Part model, mm, in its own coordinate system. A direction names the side the tool comes from. Round coordinates to 2 decimals unless told otherwise and drop trailing zeros. Loops run counter-clockwise (first coordinate to the right, second up) from the corner with the lowest first, then second, coordinate; pieces in that order, holes last.
(1) Cut at A-A on x = 0. List the corners of the cut face in (y, z), then the cut area to 3 significant figures.
(2) Probe probe 1 along X at (y, z) = (0, -12.5); probe 2 along Z at (x, y) = (7.6, 0). List the from-to ranges inside material, lowest first.
(3) Cut at B-B on z = -7. List the corners of the cut face in (x, y), then the cut area to 3 significant figures.
(4) Mould opens along Y. For faces 1 (the face through (7.829, 0.222, -2.875)), 2 (the face through (-1.9, 6.3, -15)), 3 (the face through (-8.82, 2.78, -7.9)) say: +Y half, -Y half, draft (parallel to the pull), parting line (faces both ways), or undercut.
(5) Tool access for faces 4 (the face through (-11.9, 3.7, 2.5)), 5 (the face through (9, -6, 0)): list every direction of +Z, -Z, +X, -X, +Y, -Y with a clear straight run to the whole face (end or side of a thin tool).
(6) Flat gauge pins, fed straight in: pin 1 (1.5 mm diameter, centred on x = 6.5, z = -6.5, fed in from +Y); pin 2 (8 mm diameter, centred on x = 7.5, z = -11, fed in from +Y); pin 3 (7 mm diameter, centred on x = 1, y = 4.5, fed in from -Z); pin 4 (0.9 mm diameter, centred on y = 0, z = -2.17, fed in from +X). Where does each tip first touch, or does it go through?
from build123d import *

# Parameters (mm, degrees)
SKETCH1_R           = 12.461427854
BASE_EXTRUDE_DEPTH  = 5
SKETCH2_R           = 9.246210184
BOSS_EXTRUDE1_DEPTH = 15
SKETCH3_W           = 6.4135
SKETCH3_H           = 13.726679844
SKETCH4_W           = 2.875338505
SKETCH4_H           = 0.738225097
SKETCH5_W           = 2.875338506
SKETCH5_H           = 0.738225097
FILLET1_R           = 1


with BuildPart() as part:
    # Sketch1 → Base-Extrude (new body)
    with BuildSketch(Plane(origin=(0, 0, 0), x_dir=(-1, 0, 0), z_dir=(0, 0, -1))):
        Circle(SKETCH1_R)
    extrude(amount=-BASE_EXTRUDE_DEPTH)

    # Sketch2 → Boss-Extrude1 (add)
    with BuildSketch(Plane(origin=(0, 0, 0), x_dir=(-1, 0, 0), z_dir=(0, 0, -1))):
        Circle(SKETCH2_R)
    extrude(amount=BOSS_EXTRUDE1_DEPTH)

    # Sketch3 → Cut-Revolve1 (revolve, cut)
    with BuildSketch(Plane.XZ):
        with Locations((3.20675, -8.136660078)):
            Rectangle(SKETCH3_W, SKETCH3_H)
    revolve(axis=Axis((0, 0, -1.273320156), (0, 0, -1)), mode=Mode.SUBTRACT)

    # Sketch4 → Cut-Revolve2 (revolve, cut)
    with BuildSketch(Plane(origin=(0, 0, 0), x_dir=(1, 0, 0), z_dir=(0, 1, 0))):
        with Locations((-7.808540932, 2.539892603)):
            Rectangle(SKETCH4_W, SKETCH4_H)
    revolve(axis=Axis((-9.246210184, 0, -2.170780054), (1, 0, 0)), mode=Mode.SUBTRACT)

    # Sketch5 → Cut-Revolve3 (revolve, cut)
    with BuildSketch(Plane(origin=(0, 0, 0), x_dir=(1, 0, 0), z_dir=(0, 1, 0))):
        with Locations((7.808540932, 2.539892603)):
            Rectangle(SKETCH5_W, SKETCH5_H)
    revolve(axis=Axis((6.370871679, 0, -2.170780054), (1, 0, 0)), mode=Mode.SUBTRACT)

    # Fillet1
    fillet1_edges = [part.edges().sort_by_distance(p)[0] for p in [
        (12.461427854, 0, 0),
        (12.461427854, 0, 5),
        (9.246210184, 0, 0),
    ]]
    fillet(fillet1_edges, radius=FILLET1_R)


solid = part.part
Final values:
1. outline: (-12.46, 1) arc R1 ccw to (-11.46, 0) - (-10.25, 0) arc R1 cw to (-9.25, -1) - (-9.25, -15) - (-6.41, -15) - (-6.41, -1.27) - (6.41, -1.27) - (6.41, -15) - (9.25, -15) - (9.25, -1) arc R1 cw to (10.25, 0) - (11.46, 0) arc R1 ccw to (12.46, 1) - (12.46, 4) arc R1 ccw to (11.46, 5) - (-11.46, 5) arc R1 ccw to (-12.46, 4) - close
1. area: 225 mm2
2. probe 1: x = -9.25 to -6.41, 6.41 to 9.25
2. probe 2: z = -15 to -2.91, -1.43 to 5
3. outline: circle Ø18.49 at (0, 0); hole circle Ø12.83 at (0, 0)
3. area: 139 mm2
4. face 1: undercut
4. face 2: draft
4. face 3: parting line
5. face 4: +Z, -Z
5. face 5: -Z
6. pin 1: stops at y = 7.24
6. pin 2: stops at y = 8.56
6. pin 3: stops at z = -15
6. pin 4: passes through
